Job drawing, mm, ordinate dimensions from the low corner. One solid piece. Give positions to 0.01 mm unless a question says otherwise; leave off trailing zeros. Order: outer loops, then holes, each group sorted by start corner. A loop starts at its lowest first (then second) coordinate and runs counter-clockwise, first axis right, second up. Notation, with made-up numbers: M -3.5,17 L 48.5,17 A20 ccw 48.5,29 Z; hole C -17,77.5 d3. An arc over 180 degrees is marked long. One line per question, with ' | ' between items.
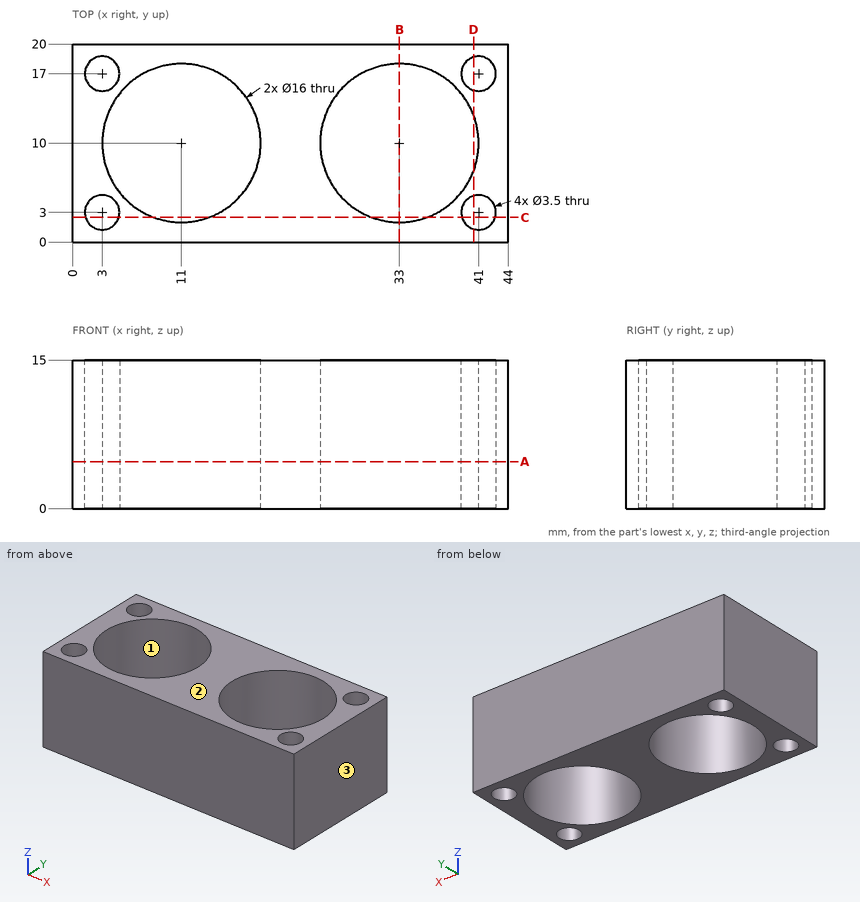
1. Slice it at C-C on y = 2.5. Give the cut face in (x, z).
Worked out:
outline: M 0,0 L 1.32,0 L 1.32,15 L 0,15 Z; M 4.68,0 L 8.22,0 L 8.22,15 L 4.68,15 Z; M 13.78,0 L 30.22,0 L 30.22,15 L 13.78,15 Z; M 35.78,0 L 39.32,0 L 39.32,15 L 35.78,15 Z; M 42.68,0 L 44,0 L 44,15 L 42.68,15 Z
2. Slice it at A-A on z = 4.75. Give the cut face in (x, y), then the cut area to 3 significant figures.
Worked out:
outline: M 0,0 L 44,0 L 44,20 L 0,20 Z; hole C 3,3 d3.5; hole C 3,17 d3.5; hole C 11,10 d16; hole C 33,10 d16; hole C 41,3 d3.5; hole C 41,17 d3.5 | area: 439 mm2
3. Slice it at D-D on x = 40.5. Give the cut face in (y, z), then the cut area to 3 significant figures.
Worked out:
outline: M 0,0 L 1.32,0 L 1.32,15 L 0,15 Z; M 4.68,0 L 7.22,0 L 7.22,15 L 4.68,15 Z; M 12.78,0 L 15.32,0 L 15.32,15 L 12.78,15 Z; M 18.68,0 L 20,0 L 20,15 L 18.68,15 Z | area: 116 mm2
4. Mould opens along X. For the marked faces 1, 2 and 3 say: released by +X, released by -X, zero draft, split by the parting line, or undercut.
Worked out:
face 1: undercut | face 2: zero draft | face 3: released by +X
5. Slice it at B-B on x = 33. Give the cut face in (y, z).
Worked out:
outline: M 0,0 L 2,0 L 2,15 L 0,15 Z; M 18,0 L 20,0 L 20,15 L 18,15 Z
6. Probe L1, parallel to Y at x = 33, z = 6.75; L2, parallel to X at y = 9.75, z = 11.25; L3, parallel to X at y = 14, z = 13.25. List the from-to ranges inside material, lowest first. Write a range as from..to.
Worked out:
L1: y = 0..2, 18..20 | L2: x = 0..3, 19..25, 41..44 | L3: x = 0..4.07, 17.93..26.07, 39.93..44
7. Drop a flat-ended pin along its axis: pin 1 (3 mm diameter, centred on x = 3, y = 3, fed in from -Z). Give the stop position or say it passes through.
Worked out:
pin 1: passes through
